from build123d import *

# Parameters (mm, degrees)
BOSS_EXTRUDE1_DEPTH = 25.4
SCALE1_SCALE        = 25.365591398
SKETCH3_W           = 1042.369657432
SKETCH3_H           = 1273.252838884
CUT_EXTRUDE1_DEPTH  = 618.998
CHAMFER1_SIZE       = 50.8
CHAMFER2_SIZE       = 38.1
CHAMFER3_SIZE       = 40.64
CHAMFER3_SIZE2      = 40.894583593
CHAMFER4_SIZE       = 40.64
CHAMFER4_SIZE2      = 41.405123541
SKETCH4_W           = 25.4
SKETCH4_H           = 106.871356521
CUT_EXTRUDE2_DEPTH  = 618.998
SKETCH5_W           = 76.2
SKETCH5_H           = 25.4
CUT_EXTRUDE3_DEPTH  = 800.296261243
LPATTERN4_COUNT     = 2
LPATTERN4_PITCH     = 106.68
CUT_EXTRUDE4_DEPTH  = 25.4


with BuildPart() as part:
    # Sketch1 → Boss-Extrude1 (new body)
    with BuildSketch(Plane.XY):
        Polygon((-15.617276252, -25), (-13.194626522, -25), (-12.617276252, -24), (8.382723748, -24), (8.960074017, -25), (11.382723748, -25), (11.382723748, -21.02978992), (-9.117276252, 17.18), (-9.117276252, 22.18), (-15.617276252, 22.18), (-15.617276252, -18.433701616), (-17.522276252, -19.533553879), (-17.522276252, -21.733258405), (-15.617276252, -22.833110667), align=None)
        Polygon((-12.617276252, -20), (7.425731864, -20), (-2.548020957, -1.41), (-12.617276252, -1.41), align=None, mode=Mode.SUBTRACT)
    extrude(amount=BOSS_EXTRUDE1_DEPTH)


with BuildPart() as part_1:
    # Scale1: scaled about (-6.821956607, -3.861646577, 12.7)
    add(part.part.scale(SCALE1_SCALE).moved(Location((166.22100722, 94.091302618, -309.443010753))))

    # Sketch3 → Cut-Extrude1 (cut)
    with BuildSketch(Plane(origin=(0, 0, -309.443010753), x_dir=(-1, 0, 0), z_dir=(0, 0, -1))):
        with Locations((-113.67141854, 36.826872795)):
            Rectangle(SKETCH3_W, SKETCH3_H)
    extrude(amount=-CUT_EXTRUDE1_DEPTH, mode=Mode.SUBTRACT)

    # Chamfer1
    chamfer1_edges = [part_1.edges().sort_by_distance(p)[0] for p in [
        (-65.044096862, 656.700119822, 322.199),
    ]]
    chamfer(chamfer1_edges, length=CHAMFER1_SIZE)

    # Chamfer2
    chamfer2_edges = [part_1.edges().sort_by_distance(p)[0] for p in [
        (-153.823666755, -413.220525339, 322.199),
        (-153.823666755, 58.325818747, 322.199),
    ]]
    chamfer(chamfer2_edges, length=CHAMFER2_SIZE)

    # Chamfer3
    chamfer3_edges = [part_1.edges().sort_by_distance(p)[0] for p in [
        (101.588948743, 58.325818747, 322.199),
    ]]
    chamfer3_side = [part_1.faces().sort_by_distance(p)[0] for p in [
        (-7.067359006, 58.325818747, 322.199),
    ]]
    chamfer(chamfer3_edges, length=CHAMFER3_SIZE, length2=CHAMFER3_SIZE2, reference=chamfer3_side[0])

    # Chamfer4
    chamfer4_edges = [part_1.edges().sort_by_distance(p)[0] for p in [
        (354.579087503, -413.220525339, 322.199),
    ]]
    chamfer4_side = [part_1.faces().sort_by_distance(p)[0] for p in [
        (237.750829348, -195.465247251, 322.199),
    ]]
    chamfer(chamfer4_edges, length=CHAMFER4_SIZE, length2=CHAMFER4_SIZE2, reference=chamfer4_side[0])

    # Sketch4 → Cut-Extrude2 (cut)
    with BuildSketch(Plane.XY.offset(334.843010753)):
        with Locations((-227.077270504, -486.612804068)):
            Rectangle(SKETCH4_W, SKETCH4_H)
    extrude(amount=-CUT_EXTRUDE2_DEPTH, mode=Mode.SUBTRACT)

    # Sketch5 → Cut-Extrude3 (cut, through all)
    with BuildSketch(Plane.XY.offset(334.843010753)):
        with Locations((-153.322884144, 323.297517672)):
            Rectangle(SKETCH5_W, SKETCH5_H)
        with Locations((-153.322884144, 216.617517672)):
            Rectangle(SKETCH5_W, SKETCH5_H)
        with Locations((-153.322884144, 429.977517672)):
            Rectangle(SKETCH5_W, SKETCH5_H)
        with Locations((-153.322884144, 376.637517672)):
            Rectangle(SKETCH5_W, SKETCH5_H)
        with Locations((-153.322884144, 269.957517672)):
            Rectangle(SKETCH5_W, SKETCH5_H)
        with Locations((-153.322884144, 163.277517672)):
            Rectangle(SKETCH5_W, SKETCH5_H)
        with Locations((-153.322884144, 109.937517672)):
            Rectangle(SKETCH5_W, SKETCH5_H)
    cut_extrude3 = extrude(amount=-CUT_EXTRUDE3_DEPTH, mode=Mode.SUBTRACT)

    # LPattern4: Cut-Extrude3 ×2
    with Locations(*[(0, i * LPATTERN4_PITCH, 0) for i in range(1, LPATTERN4_COUNT)]):
        add(cut_extrude3, mode=Mode.SUBTRACT)

    # Sketch6 → Cut-Extrude4 (cut)
    with BuildSketch(Plane.ZY.offset(214.377270504)):
        Polygon((334.843010753, -433.177125807), (309.554989247, -433.177125807), (334.843010753, -411.957956289), align=None)
    extrude(amount=CUT_EXTRUDE4_DEPTH, mode=Mode.SUBTRACT)


solid = part_1.part
CAD build for the part. Positions are in the model's coordinates, mm. A direction names the side the tool comes from. Round coordinates to 2 decimals unless told otherwise and drop trailing zeros. Write each loop counter-clockwise with the first axis right and the second up, starting at its lowest first coordinate (ties: lowest second). Pieces come first, ordered by that corner, then holes. Notation, with made-up numbers: M -29,31.5 L -5,31.5 A10 ccw -5,45.5 Z; hole C 57,30 d4. An arc over 180 degrees is marked long. Use a Markdown table: item, result. Add a question column.
1. Slice it at A-A on x = -85.5. Give the cut face in (y, z), then the cut area to 3 significant figures.
2. Slice it at D-D on y = 244. Give the cut face in (x, z), then the cut area to 3 significant figures.
3. Slice it at B-B on y = -223. Give the cut face in (x, z), then the cut area to 3 significant figures.
4. 3-axis set-ups, long thin cutter, end or side, ignore diameter. For faces 1 (the face through (2, 67, 334.843)), 2 (the face through (109, -514.683, 322)), 3 (the face through (-154, 257.258, 322)): which of +Z, -Z, +X, -X, +Y, -Y reach the whole face in a straight line?
5. Flat gauge pins, fed straight in: P1, Ø2, axis at x = -103, z = 313.5, coming from the -Y side; P2, Ø12.5, axis at y = 210.5, z = 321.5, coming from the +X side; P3, Ø10, axis at y = 233.5, z = 313, coming from the -X side. Where does each tip first touch, or does it go through?
6. Pull direction Y, two halves, no side cores. Call faces 4 (the face through (-278.242, -429, 322)), 5 (the face through (-115.223, 376, 322)), 6 (the face through (-253.743, -387.244, 322.022)): released by +Y, released by -Y, zero draft, split by the parting line, or undercut.
7. Drill centre lines: probe 1 along X at (y, z) = (418.5, 321.5); probe 2 along X at (y, z) = (333.5, 315.25); probe 3 along Y at (x, z) = (-82, 324). Where is each one in solid material? Low to high.
8. Slice it at C-C on z = 318.25. Give the number of separate pieces and of enclosed holes in the cut face, then the cut area to 3 significant figures.
Reply:
| question | item | result |
|---|---|---|
| 1 | outline | M -514.68,309.55 L -413.22,309.55 L -413.22,334.84 L -514.68,334.84 Z; M 58.33,309.55 L 626.36,309.55 L 626.36,334.84 L 58.33,334.84 Z |
| 1 | area | 16,900 mm^2 |
| 2 | outline | M -229.92,309.55 L 88.33,309.55 L 88.33,334.84 L -229.92,334.84 Z |
| 2 | area | 8,050 mm^2 |
| 3 | outline | M -229.92,309.55 L -153.82,309.55 L -153.82,334.84 L -229.92,334.84 Z; M 252.52,309.55 L 338.88,309.55 L 338.88,334.84 L 252.52,334.84 Z |
| 3 | area | 4,110 mm^2 |
| 4 | face 1 | +Z, +X, -X, +Y, -Y |
| 4 | face 2 | +Z, -Z, -Y |
| 4 | face 3 | +Z, -Z |
| 5 | P1 | stops at y = -514.68 |
| 5 | P2 | stops at x = 109.66 |
| 5 | P3 | stops at x = -229.92 |
| 6 | face 4 | zero draft |
| 6 | face 5 | undercut |
| 6 | face 6 | released by +Y |
| 7 | probe 1 | x = -229.92 to -191.42, -115.22 to -5.29 |
| 7 | probe 2 | x = -229.92 to -191.42, -115.22 to 40.31 |
| 7 | probe 3 | y = -514.68 to -413.22, 58.33 to 622.86 |
| 8 | separate pieces | 1 |
| 8 | enclosed holes | 10 |
| 8 | area | 294,000 mm^2 |
